```python
from build123d import *

# Parameters (mm, degrees)
SKETCH1_W           = 12
SKETCH1_H           = 15
BOSS_EXTRUDE1_DEPTH = 20
SKETCH2_R           = 1.6
BOSS_EXTRUDE2_DEPTH = 5
SKETCH3_R           = 1.6
CUT_EXTRUDE1_DEPTH  = 10
CUT_EXTRUDE2_DEPTH  = 3
CUT_EXTRUDE3_DEPTH  = 2
BOSS_EXTRUDE4_DEPTH = 3.7
BOSS_EXTRUDE5_START = -5
SKETCH8_W           = 2.336067977
SKETCH8_H           = 8.6
BOSS_EXTRUDE5_DEPTH = 5
SKETCH10_W          = 15
SKETCH10_H          = 5.4
CUT_EXTRUDE5_DEPTH  = 7
BOSS_EXTRUDE8_START = -5
SKETCH13_W          = 2.336067977
SKETCH13_H          = 5.4
BOSS_EXTRUDE8_DEPTH = 5


with BuildPart() as part:
    # Sketch1 → Boss-Extrude1 (new body)
    with BuildSketch(Plane(origin=(0, 0, 0), x_dir=(1, 0, 0), z_dir=(0, 1, 0))):
        Rectangle(SKETCH1_W, SKETCH1_H)
    extrude(amount=BOSS_EXTRUDE1_DEPTH)

    # Sketch2 → Boss-Extrude2 (add)
    # profile 1 of 2: a face of its own
    with BuildSketch(Plane.ZY.offset(6)):
        with BuildLine():
            Line((10.5, 11.4), (7.5, 11.4))
            Line((7.5, 11.4), (7.5, 5.4))
            Line((7.5, 5.4), (10.5, 5.4))
            ThreePointArc((10.5, 5.4), (13.5, 8.4), (10.5, 11.4))
        make_face()
        with Locations((10.5, 8.4)):
            Circle(SKETCH2_R, mode=Mode.SUBTRACT)
    # profile 2 of 2: a face of its own
    with BuildSketch(Plane.ZY.offset(6)):
        with BuildLine():
            Line((-10.5, 11.4), (-7.5, 11.4))
            Line((-7.5, 11.4), (-7.5, 5.4))
            Line((-7.5, 5.4), (-10.5, 5.4))
            ThreePointArc((-10.5, 5.4), (-13.5, 8.4), (-10.5, 11.4))
        make_face()
        with Locations((-10.5, 8.4)):
            Circle(SKETCH2_R, mode=Mode.SUBTRACT)
    extrude(amount=-BOSS_EXTRUDE2_DEPTH)

    # Sketch3 → Cut-Extrude1 (cut)
    with BuildSketch(Plane(origin=(0, 20, 0), x_dir=(1, 0, 0), z_dir=(0, 1, 0))):
        with Locations(Location((-1, 0, 0), (0, 0, 270))):
            Circle(SKETCH3_R)
    extrude(amount=-CUT_EXTRUDE1_DEPTH, mode=Mode.SUBTRACT)

    # Sketch4 → Cut-Extrude2 (cut)
    with BuildSketch(Plane(origin=(0, 18, 0), x_dir=(1, 0, 0), z_dir=(0, 1, 0))):
        Polygon((-2.674315781, 2.9), (-6, 2.9), (-6, -2.9), (-2.674315781, -2.9), (0.674315781, -2.9), (2.348631561, 0), (0.674315781, 2.9), align=None)
    extrude(amount=-CUT_EXTRUDE2_DEPTH, mode=Mode.SUBTRACT)

    # Sketch5 → Cut-Extrude3 (cut)
    with BuildSketch(Plane(origin=(0, 18, 0), x_dir=(1, 0, 0), z_dir=(0, 1, 0))):
        with BuildLine():
            Line((-1, 1.8), (6, 2))
            Line((6, 2), (6, 0))
            Line((6, 0), (6, -2))
            Line((6, -2), (-1, -1.8))
            ThreePointArc((-1, -1.8), (-2.8, 0), (-1, 1.8))
        make_face()
    extrude(amount=CUT_EXTRUDE3_DEPTH, mode=Mode.SUBTRACT)

    # Sketch6 → Boss-Extrude4 (add)
    with BuildSketch(Plane(origin=(0, 20, 0), x_dir=(1, 0, 0), z_dir=(0, 1, 0))):
        Polygon((-6, 7.7), (-6, 7.5), (-1, 7.5), (-1, 9.836067977), (-8, 9.836067977), (-8, 7.7), align=None)
        Polygon((-1, -7.5), (-6, -7.5), (-6, -7.7), (-8, -7.7), (-8, -9.836067977), (-1, -9.836067977), align=None)
    extrude(amount=-BOSS_EXTRUDE4_DEPTH)

    # Sketch8 → Boss-Extrude5 (add)
    with BuildSketch(Plane(origin=(-1, 0, 0), x_dir=(0, 0, -1), z_dir=(1, 0, 0)).offset(BOSS_EXTRUDE5_START)):
        with Locations((-8.668033989, 15.7)):
            Rectangle(SKETCH8_W, SKETCH8_H)
        with Locations((8.668033989, 15.7)):
            Rectangle(SKETCH8_W, SKETCH8_H)
    extrude(amount=BOSS_EXTRUDE5_DEPTH)

    # Sketch10 → Cut-Extrude5 (cut)
    with BuildSketch(Plane(origin=(6, 0, 0), x_dir=(0, 0, -1), z_dir=(1, 0, 0))):
        with Locations((0, 2.7)):
            Rectangle(SKETCH10_W, SKETCH10_H)
    extrude(amount=-CUT_EXTRUDE5_DEPTH, mode=Mode.SUBTRACT)

    # Sketch13 → Boss-Extrude8 (add)
    with BuildSketch(Plane(origin=(-1, 0, 0), x_dir=(0, 0, -1), z_dir=(1, 0, 0)).offset(BOSS_EXTRUDE8_START)):
        with Locations((8.668033989, 2.7)):
            Rectangle(SKETCH13_W, SKETCH13_H)
        with Locations((-8.668033989, 2.7)):
            Rectangle(SKETCH13_W, SKETCH13_H)
    extrude(amount=BOSS_EXTRUDE8_DEPTH)


solid = part.part
```
The model under review builds one solid part; all positions refer to its coordinate system, in mm. A direction names the side the tool comes from. Round coordinates to 2 decimals unless told otherwise and drop trailing zeros. Loops run counter-clockwise (first coordinate to the right, second up) from the corner with the lowest first, then second, coordinate; pieces in that order, holes last. Notation, with made-up numbers: (62.25, 24) - (105.25, 24) arc R16 ccw to (105.25, 47) - close; hole circle Ø1 at (32.5, 50.5). An arc over 180 degrees is marked (long way). Use a Markdown table: item, result. Add a question column.
Q1. Insertion check: pin 1 Ø7.5 at (x, y) = (2.5, 11) entering from +Z; pin 2 Ø0.5 at (x, z) = (-3, -10) entering from +Y; pin 3 Ø4 at (x, y) = (-3.5, 12) entering from +Z; pin 4 Ø1.5 at (x, y) = (-3, 16) entering from +Z. Each pin has a flat end and moves straight along its axis. Give the tip position at first contact, or say it passes through.
Q2. The part is to be moulded in two halves that separate along Z. For faces 4 (the face through (-3.54, 8.47, 8.9)), 5 (the face through (2, 13, 7.5)), 6 (the face through (-4, 16, -9.836)), say which applies: pulls with the +Z half, pulls with the -Z half, needs draft (parallel to the pull), parting line crosses it, or undercut.
Q3. Add section B-B (y = 8.4). State the section outline as (x, z) points, plus the area to 3 significant figures.
Q4. Add section D-D (z = 11.25). State the section outline as (x, y) points.
Q5. Add section C-C (y = 18.5). State the section outline as (x, z) points, plus the area to 3 significant figures.
Q6. For probe 1 along Y at (x, z) = (-4.9, 10.5); probe 2 along X at (y, z) = (12.95, 0); probe 3 along Y at (x, z) = (-5, -1.25), list the stretches that pass through material, from the lowest coordinate up.
Q7. Add section A-A (y = 12.5). State the section outline as (x, z) points.
Q8. Machinability: for faces 1 (the face through (-3, 18, 0)), 2 (the face through (-4, 16, 9.836)), 3 (the face through (2, 13, -7.5)), which of the approach directions +Z, -Z, +X, -X, +Y, -Y give a long, thin tool a straight path to every point of the face, cutting with its end or side? Answer none if there is none.
Worked answers:
| question | item | result |
|---|---|---|
| 1 | pin 1 | z = 13.23 |
| 1 | pin 2 | y = 20 |
| 1 | pin 3 | z = 13.04 |
| 1 | pin 4 | z = 9.84 |
| 2 | face 4 | undercut |
| 2 | face 5 | pulls with the +Z half |
| 2 | face 6 | pulls with the -Z half |
| 3 | outline | (-6, -13.5) - (-1, -13.5) - (-1, -12.1) - (-6, -12.1) - close; (-6, -8.9) - (-1, -8.9) - (-1, -7.5) - (6, -7.5) - (6, 7.5) - (-1, 7.5) - (-1, 8.9) - (-6, 8.9) - close; (-6, 12.1) - (-1, 12.1) - (-1, 13.5) - (-6, 13.5) - close |
| 3 | area | 208 mm² |
| 4 | outline | (-6, 5.5) - (-1, 5.5) - (-1, 6.99) - (-6, 6.99) - close; (-6, 9.81) - (-1, 9.81) - (-1, 11.3) - (-6, 11.3) - close |
| 5 | outline | (-8, -9.84) - (-1, -9.84) - (-1, -7.5) - (6, -7.5) - (6, -2) - (-1, -1.8) arc R1.8 cw to (-1, 1.8) - (6, 2) - (6, 7.5) - (-1, 7.5) - (-1, 9.84) - (-8, 9.84) - (-8, 7.7) - (-6, 7.7) - (-6, -7.7) - (-8, -7.7) - close |
| 5 | area | 180 mm² |
| 6 | probe 1 | 5.4 to 6.8, 10 to 11.4 |
| 6 | probe 2 | -6 to -2.6, 0.6 to 6 |
| 6 | probe 3 | 0 to 15, 18 to 20 |
| 7 | outline | (-6, -9.84) - (-1, -9.84) - (-1, -7.5) - (6, -7.5) - (6, 7.5) - (-1, 7.5) - (-1, 9.84) - (-6, 9.84) - close; hole circle Ø3.2 at (-1, 0) |
| 8 | face 1 | -X |
| 8 | face 2 | +Z, +X, -X, +Y |
| 8 | face 3 | -Z, +X, +Y, -Y |
